Autodesk Inventor part; units mm, degrees
ref_plane "YZ Plane" through (0, 0, 0) normal (1, 0, 0) x (0, 1, 0)
ref_plane "XZ Plane" through (0, 0, 0) normal (0, 1, 0) x (-1, 0, 0)
ref_plane "XY Plane" through (0, 0, 0) normal (0, 0, 1) x (1, 0, 0)
sketch "Sketch1" plane through (0, 0, 0) normal (0, 0, 1) x (1, 0, 0)
  arc A0 (4.5113, -11.8717) -> (6.35, -10.9985) centre (0, 0) ccw
  line L0 (6.35, 10.9985) -> (9.525, 16.4978)
  line L1 (12.7, 0) -> (19.05, 0) construction
  line L2 (10.9985, 6.35) -> (16.4978, 9.525)
  line L3 (0, 0) -> (19.05, 0) construction
  line L4 (0, 12.7) -> (0, 19.05)
  line L5 (-6.35, 10.9985) -> (-9.525, 16.4978)
  line L6 (0, 0) -> (19.05, 0) construction
  line L7 (-10.9985, 6.35) -> (-16.4978, 9.525)
  line L8 (12.7, 0) -> (26.2861, 0) construction
  line L9 (0, 0) -> (19.05, 0)
  line L10 (-12.7, 0) -> (-19.05, 0)
  line L11 (6.35, -10.9985) -> (9.525, -16.4978)
  line L12 (10.9985, -6.35) -> (16.4978, -9.525)
  line L13 (0, -12.7) -> (0, -19.05)
  line L14 (-6.35, -10.9985) -> (-9.525, -16.4978)
  line L15 (-10.9985, -6.35) -> (-16.4978, -9.525)
  arc A1 (16.4978, -9.525) -> (12.7, 0) centre (6.7257, -7.9017) ccw
  arc A2 (19.05, 0) -> (10.9985, 6.35) centre (9.7755, -3.4802) ccw
  arc A3 (16.4978, 9.525) -> (6.35, 10.9985) centre (10.2059, 1.8738) ccw
  arc A4 (9.525, 16.4978) -> (0, 12.7) centre (7.9017, 6.7257) ccw
  arc A5 (0, -19.05) -> (6.35, -10.9985) centre (-3.4802, -9.7755) ccw
  arc A6 (9.525, -16.4978) -> (10.9985, -6.35) centre (1.8738, -10.2059) ccw
  arc A7 (0, 19.05) -> (-6.35, 10.9985) centre (3.4802, 9.7755) ccw
  arc A8 (-9.525, 16.4978) -> (-10.9985, 6.35) centre (-1.8738, 10.2059) ccw
  arc A9 (-9.525, -16.4978) -> (0, -12.7) centre (-7.9017, -6.7257) ccw
  arc A10 (-16.4978, -9.525) -> (-6.35, -10.9985) centre (-10.2059, -1.8738) ccw
  arc A11 (-19.05, 0) -> (-10.9985, -6.35) centre (-9.7755, 3.4802) ccw
  arc A12 (-16.4978, 9.525) -> (-12.7, 0) centre (-6.7257, 7.9017) ccw
  dimension "d0" = 25.4
  dimension "d1" = 19.05
  dimension "d2" = 60
  dimension "d3" = 19.05
  dimension "d4" = 30
  dimension "d5" = 19.05
  dimension "d6" = 120
  dimension "d7" = 150
  dimension "d8" = 9.906
  dimension "d9" = 9.906
  dimension "d10" = 9.906
  dimension "d11" = 9.906
  dimension "d18" = 9.906
  dimension "d19" = 9.906
  dimension "d20" = 9.906
  dimension "d21" = 9.906
  dimension "d22" = 9.906
  dimension "d23" = 9.906
  dimension "d24" = 9.906
  dimension "d25" = 9.906
extrude "Extrusion1" add sketch "Sketch1" along normal blind 12.7
sketch "Sketch2" plane through (0, 0, 12.7) normal (0, 0, 1) x (1, 0, 0)
  circle A0 centre (0, 0) radius 2.54
  dimension "d28" = 5.08
extrude "Extrusion2" cut sketch "Sketch2" against normal blind 12.7
properties part number "ratchet prototype"
Could you check a few things on this model? Use its own coordinates, in mm. A direction names the side the tool comes from. Round coordinates to 2 decimals unless told otherwise and drop trailing zeros. Loops run counter-clockwise (first coordinate to the right, second up) from the corner with the lowest first, then second, coordinate; pieces in that order, holes last. Notation, with made-up numbers: (63, 44.5) -> (106, 44.5) arc R28 cw to (106, 64.5) -> close; hole circle Ø7 at (87, 62). An arc over 180 degrees is marked (long way). Put each result on its own line as item: value.
Q1. Which directions (+Z, -Z, +X, -X, +Y, -Y) give clear straight access to the entire face, cutting with the end or side of a thin tool? Please do faces 1 (the flat face through (0, 5, 0)), 2 (the flat face through (-16, 0, 6)), 3 (the flat face through (16, 0, 6)).
Checks:
face 1: -Z, +X, -X, +Y, -Y
face 2: +Z, -Z, -X
face 3: +Z, -Z, +X
Q2. For pin 1 Ø4.5 at (x, y) = (0, 0) entering from -Z; pin 2 Ø1 at (x, z) = (14, 4.5) entering from -Y; pin 3 Ø5 at (y, z) = (3.5, 5.5) entering from -X; pin 4 Ø1 at (x, z) = (5, 3) entering from +Y, each with a flat end and sliding along its axis, tell me the tip position at first contact or that it passes through.
Checks:
pin 1: through
pin 2: y = -8.37
pin 3: x = -16.45
pin 4: y = 16.34
Q3. I want a section at B-B on x = -7.5. Write out the boundary of the cut face in (y, z).
Checks:
outline: (-16.62, 0) -> (-12.99, 0) -> (-12.99, 12.7) -> (-16.62, 12.7) -> close; (-11.4, 0) -> (12.99, 0) -> (12.99, 12.7) -> (-11.4, 12.7) -> close
Q4. I want a section at C-C on y = -13.5. Write out the boundary of the cut face in (x, z).
Checks:
outline: (-7.79, 0) -> (-0.67, 0) -> (-0.67, 12.7) -> (-7.79, 12.7) -> close; (0, 0) -> (5.7, 0) -> (5.7, 12.7) -> (0, 12.7) -> close; (7.79, 0) -> (11.22, 0) -> (11.22, 12.7) -> (7.79, 12.7) -> close
Q5. Please list where these lines run through material, in increasing order: line 1 (X direction, y = 14, z = 6.25); line 2 (Y direction, x = 13, z = 9.25); line 3 (X direction, y = 1, z = 4.75). Write a range as from..to.
Checks:
line 1: -11.02..-8.08, -5.48..0, 1.18..8.08
line 2: -7.51..-0.24, 0..5.89, 7.51..11.38
line 3: -13.83..-2.33, 2.33..18.61
Q6. Thinking about a two-plate mould opening in Y: for faces 4 (the cylindrical face through (-0.33, 2.52, 6.44)), 5 (the cylindrical face through (11.55, 11.69, 6.26)), 6 (the flat face through (-7.915, 13.71, 6.261)), 7 (the flat face through (0, 16, 6)), which applies, pulls with the +Y half, pulls with the -Y half, needs draft (parallel to the pull), parting line crosses it, or undercut?
Checks:
face 4: undercut
face 5: undercut
face 6: pulls with the +Y half
face 7: needs draft
